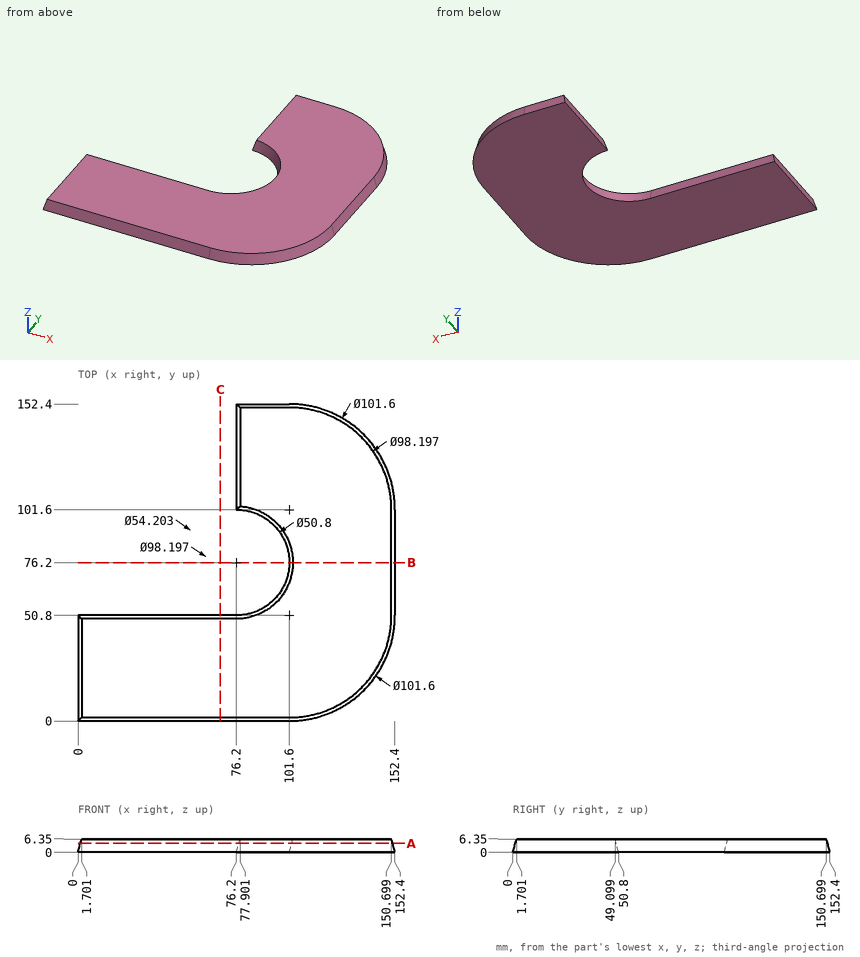
Print and shaded views of the part. All mm, measured from the part's lowest x, y and z. Give positions to 0.01 mm unless a question says otherwise; leave off trailing zeros. Loops run counter-clockwise (first coordinate to the right, second up) from the corner with the lowest first, then second, coordinate; pieces in that order, holes last. Notation, with made-up numbers: (-27.75, 37.25) - (-2.75, 37.25) arc R27 cw to (-2.75, 72.25) - close; hole circle Ø10 at (41.5, 56). An arc over 180 degrees is marked (long way). Use a Markdown table: item, result.
(1) Band-saw the part on B-B (y = 76.2). Give the cut face in (x, z).
Taken from the geometry:
| item | result |
|---|---|
| outline | (101.6, 0) - (152.4, 0) - (150.7, 6.35) - (103.3, 6.35) - close |
(2) Wall check: line 1 along Y through (x, z) = (87.5, 3.25) (1 decimal); line 2 along X through (y, z) = (54.5, 1.25) (1 decimal); line 3 along X through (y, z) = (140.5, 3.5) (1 decimal). Give the ranges that are in metal, low to high.
Taken from the geometry:
| item | result |
|---|---|
| line 1 | 0.9 to 52.5, 99.9 to 151.5 |
| line 2 | 90 to 152.1 |
| line 3 | 77.1 to 132.8 |
(3) Band-saw the part on C-C (x = 68.5). Give the cut face in (y, z), and give its area (3 significant figures).
Taken from the geometry:
| item | result |
|---|---|
| outline | (0, 0) - (50.8, 0) - (49.1, 6.35) - (1.7, 6.35) - close |
| area | 312 mm2 |
(4) Band-saw the part on A-A (z = 4.25). Give the cut face in (x, y) (1 decimal), and give its area (3 significant figures).
Taken from the geometry:
| item | result |
|---|---|
| outline | (1.1, 1.1) - (101.6, 1.1) arc R49.7 ccw to (151.3, 50.8) - (151.3, 101.6) arc R49.7 ccw to (101.6, 151.3) - (77.3, 151.3) - (77.3, 102.7) arc R26.5 cw to (76.2, 49.7) - (1.1, 49.7) - close |
| area | 12,700 mm2 |
(5) Drop flat-ended pins along their axis: pin 1 Ø1 at (y, z) = (64, 1.5) entering from +X; pin 2 Ø2 at (x, z) = (106.5, 3) entering from -Y; pin 3 Ø1 at (y, z) = (130, 2.5) entering from +X (1 decimal). Give the stop position or say it passes through.
Taken from the geometry:
| item | result |
|---|---|
| pin 1 | x = 152.13 |
| pin 2 | y = 0.76 |
| pin 3 | x = 143.3 |
